Design review of the part shown in the three views and the two pictorial views. Dimensions are in mm from the part's minimum x, y and z. A direction names the side the tool comes from. Coordinates: 2 decimals unless noted, no trailing zeros. Loops run counter-clockwise (first coordinate to the right, second up) from the corner with the lowest first, then second, coordinate; pieces in that order, holes last. Notation, with made-up numbers: M -15,-14.75 L 11,-14.75 A11 cw 11,-9.75 Z; hole C 39.25,59.25 d1. An arc over 180 degrees is marked long. Put each result on its own line as item: value. Start each with the question number.
(1) Clearance check with flat-ended pins moving along their axes: pin 1 (1.6 mm diameter, centred on x = 8, y = 6.5, fed in from +Z); pin 2 (3 mm diameter, centred on y = 8, z = 7.5, fed in from -X); pin 3 (2 mm diameter, centred on x = 6.5, y = 8, fed in from -Z); pin 4 (3 mm diameter, centred on x = 13.5, y = 7.5, fed in from +Z). State where each tip first meets the part, or that it passes through.
(2) The part is to be moulded in two halves that separate along X. For the marked faces 1, 2, 3 and 4, say which applies: +X half, -X half, draft (parallel to the pull), parting line (faces both ways), or undercut.
(3) For the marked faces 5, 6 and 7, list the 3-axis set-ups (+Z, -Z, +X, -X, +Y, -Y) from which the entire face can be reached by the end or side of a thin tool; tool diameter is ignored.
(4) Take a section at C-C, the plane z = 9.5. Give the boundary of the cut face in (x, y).
(5) Take a section at B-B, the plane x = 9.5. Give the boundary of the cut face in (y, z).
(6) Take a section at D-D, the plane y = 8. Give the boundary of the cut face in (x, z).
(7) For probe 1 along X at (y, z) = (1.5, 8); probe 2 along Z at (x, y) = (7, 1.25); probe 3 along Y at (x, z) = (5.25, 12.5), list the stretches that pass through material, from the lowest coordinate up. Write a range as [from, to].
(8) Take a section at A-A, the plane y = 1.5. Give the boundary of the cut face in (x, z).
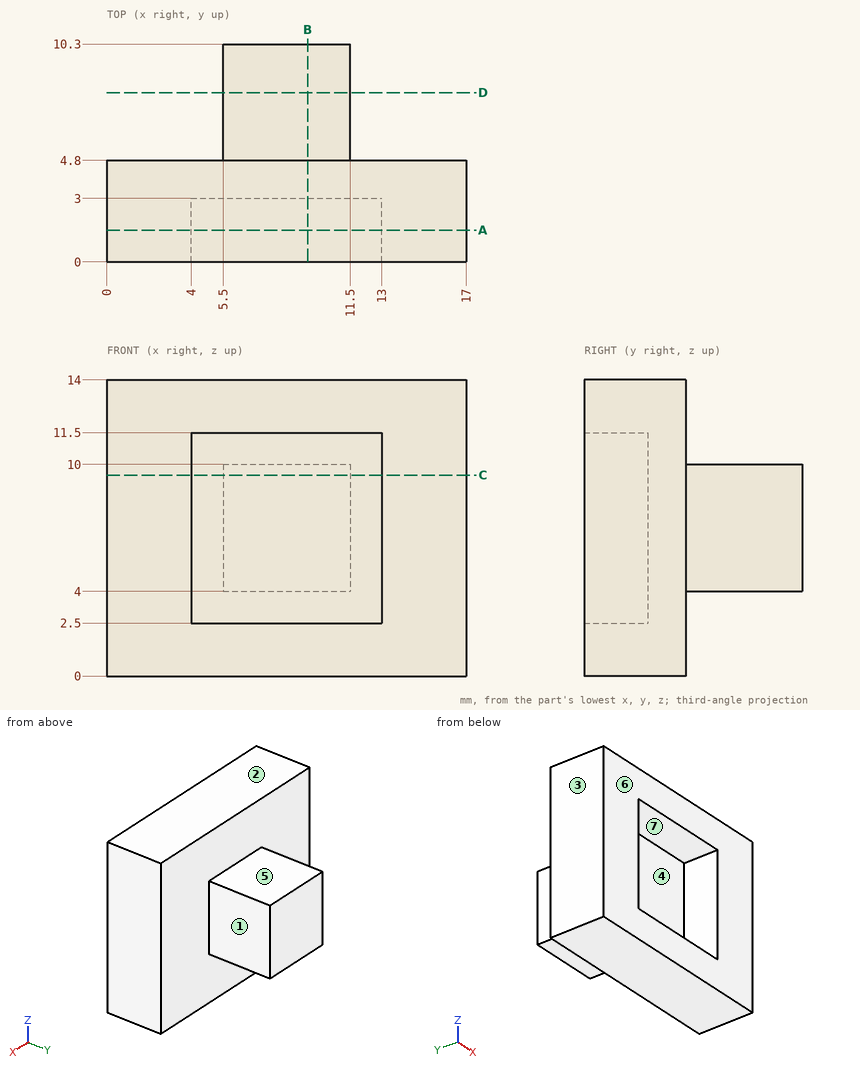
Computed values:
1. pin 1: stops at z = 10
1. pin 2: stops at x = 5.5
1. pin 3: stops at z = 4
1. pin 4: passes through
2. face 1: +X half
2. face 2: draft
2. face 3: -X half
2. face 4: undercut
3. face 5: +Z, +X, -X, +Y
3. face 6: +Z, -Z, +X, -X, -Y
3. face 7: -Y
4. outline: M 0,0 L 4,0 L 4,3 L 13,3 L 13,0 L 17,0 L 17,4.8 L 11.5,4.8 L 11.5,10.3 L 5.5,10.3 L 5.5,4.8 L 0,4.8 Z
5. outline: M 0,0 L 4.8,0 L 4.8,4 L 10.3,4 L 10.3,10 L 4.8,10 L 4.8,14 L 0,14 L 0,11.5 L 3,11.5 L 3,2.5 L 0,2.5 Z
6. outline: M 5.5,4 L 11.5,4 L 11.5,10 L 5.5,10 Z
7. probe 1: x = [0, 4], [13, 17]
7. probe 2: z = [0, 2.5], [11.5, 14]
7. probe 3: y = [0, 4.8]
8. outline: M 0,0 L 17,0 L 17,14 L 0,14 Z; hole M 4,2.5 L 13,2.5 L 13,11.5 L 4,11.5 Z
